The listing builds one solid part. Answer for the finished solid, in the listing's coordinates (mm). A direction names the side the tool comes from. Round coordinates to 2 decimals unless told otherwise and drop trailing zeros. Write each loop counter-clockwise with the first axis right and the second up, starting at its lowest first coordinate (ties: lowest second). Pieces come first, ordered by that corner, then holes. Notation, with made-up numbers: (-26.75, 82) - (17.25, 82) arc R19 ccw to (17.25, 99) - close; hole circle Ø9 at (-11.75, -31). An arc over 180 degrees is marked (long way). Return JSON: item names as keys, results as strings. Group by question number.
(1) Which of the six approach directions +Z, -Z, +X, -X, +Y, -Y give full straight-line access (tool end or side, diameter ignored) to faces 4 (the cylindrical face through (-17.281, 62.225, 6.084)), 5 (the flat face through (-20, -80, 7.9))?
(2) Section C-C, the plane x = -62 is taken. Write down the section's boundary in (y, z), then the cut area to 3 significant figures.
(3) Section B-B, the plane y = 30 is taken. Write down the section's boundary in (x, z), then the cut area to 3 significant figures.
(4) Section A-A, the plane z = 2.5 is taken. Give the number of separate pieces and of enclosed holes in the cut face, then the cut area to 3 significant figures.
(5) Each of these flat-tipped pins is pushed along its axis until it touches: pin 1 (1.5 mm diameter, centred on y = -48.5, z = 7.5, fed in from -X); pin 2 (5 mm diameter, centred on x = -19, z = 7, fed in from -Y); pin 3 (15 mm diameter, centred on x = -109.01, y = 9.57, fed in from +Z). Where does it stop, or does it pass through?
(6) Determine the mould class of faces 1 (the flat face through (-25, 8, 0)), 2 (the cylindrical face through (-22.908, 109.555, 5.916)), 3 (the cylindrical face through (51.5, 9.98, 9.04)) for opening direction Y: +Y half, -Y half, draft (parallel to the pull), parting line (faces both ways), or undercut.
(7) Find the intervals of material crossed by line 1 along X through (y, z) = (-79, 3.25); line 2 along X through (y, z) = (12, 3); line 3 along X through (y, z) = (-59, 6.5), in increasing order. Write a range as [from, to].
```python
from build123d import *

# Parameters (mm, degrees)
IZIM1_R                     = 4
Y_KSEKLIK_EKSTR_ZYON1_DEPTH = 12
IZIM2_R                     = 1.25
KES_EKSTR_ZYON1_DEPTH       = 50
KES_EKSTR_ZYON2_START       = -4.1
IZIM3_R                     = 10
IZIM3_R_2                   = 4
KES_EKSTR_ZYON2_DEPTH       = 4.1
KES_EKSTR_ZYON3_START       = -10
IZIM4_R                     = 1.35
IZIM4_R_2                   = 5.25
IZIM4_R_3                   = 4
KES_EKSTR_ZYON3_DEPTH       = 10
IZIM5_R                     = 9.5
KES_EKSTR_ZYON4_DEPTH       = 50
Y_KSEKLIK_EKSTR_ZYON2_START = -6
IZIM6_R                     = 9.5
IZIM6_R_2                   = 4.05
Y_KSEKLIK_EKSTR_ZYON2_DEPTH = 6
IZIM7_R                     = 2.6
KES_EKSTR_ZYON5_DEPTH       = 50


with BuildPart() as part:
    # Çizim1 → Yükseklik-Ekstrüzyon1 (new body)
    # profile 1 of 4: a face of its own
    with BuildSketch(Plane.XY):
        with BuildLine():
            Line((-24.007220217, 9.566787004), (-74.007220217, 59.566787004))
            ThreePointArc((-74.007220217, 59.566787004), (-124.007220217, 9.566787004), (-74.007220217, -40.433212996))
            Line((-74.007220217, -40.433212996), (-24.007220217, 9.566787004))
        make_face()
        with Locations((-109.007220217, 9.566787004)):
            Circle(IZIM1_R, mode=Mode.SUBTRACT)
    # profile 2 of 4: a face of its own
    with BuildSketch(Plane.XY):
        with BuildLine():
            ThreePointArc((25.992779783, 59.566787004), (-24.007220217, 109.566787004), (-74.007220217, 59.566787004))
            Line((-74.007220217, 59.566787004), (-24.007220217, 9.566787004))
            Line((-24.007220217, 9.566787004), (25.992779783, 59.566787004))
        make_face()
        with Locations((-24.007220217, 94.566787004)):
            Circle(IZIM1_R, mode=Mode.SUBTRACT)
    # profile 3 of 4: a face of its own
    with BuildSketch(Plane.XY):
        with BuildLine():
            Line((25.992779783, 59.566787004), (-24.007220217, 9.566787004))
            Line((-24.007220217, 9.566787004), (25.992779783, -40.433212996))
            ThreePointArc((25.992779783, -40.433212996), (75.992779783, 9.566787004), (25.992779783, 59.566787004))
        make_face()
        with Locations((60.992779783, 9.566787004)):
            Circle(IZIM1_R, mode=Mode.SUBTRACT)
    # profile 4 of 4: a face of its own
    with BuildSketch(Plane.XY):
        with BuildLine():
            Line((25.992779783, -40.433212996), (-24.007220217, 9.566787004))
            Line((-24.007220217, 9.566787004), (-74.007220217, -40.433212996))
            ThreePointArc((-74.007220217, -40.433212996), (-24.007220217, -90.433212996), (25.992779783, -40.433212996))
        make_face()
        with Locations((-24.007220217, -75.433212996)):
            Circle(IZIM1_R, mode=Mode.SUBTRACT)
    extrude(amount=Y_KSEKLIK_EKSTR_ZYON1_DEPTH)

    # Çizim2 → Kes-Ekstrüzyon1 (cut)
    with BuildSketch(Plane.XY.offset(12)):
        with Locations((-27.895001347, 40.325931985)):
            Circle(IZIM2_R)
        with Locations((-68.907194656, -0.686261324)):
            Circle(IZIM2_R)
        with Locations((-34.258962377, -35.334493602)):
            Circle(IZIM2_R)
        with Locations((6.753230931, 5.677699707)):
            Circle(IZIM2_R)
    extrude(amount=-KES_EKSTR_ZYON1_DEPTH, mode=Mode.SUBTRACT)

    # Çizim3 → Kes-Ekstrüzyon2 (cut)
    # profile 1 of 2: a face of its own
    with BuildSketch(Plane.XY.offset(12).offset(KES_EKSTR_ZYON2_START)):
        with Locations((-24.007220217, -75.433212996)):
            Circle(IZIM3_R)
        with Locations((-24.007220217, -75.433212996)):
            Circle(IZIM3_R_2, mode=Mode.SUBTRACT)
    # profile 2 of 2: a face of its own
    with BuildSketch(Plane.XY.offset(12).offset(KES_EKSTR_ZYON2_START)):
        with Locations((-24.007220217, 94.566787004)):
            Circle(IZIM3_R)
    extrude(amount=KES_EKSTR_ZYON2_DEPTH, mode=Mode.SUBTRACT)

    # Çizim4 → Kes-Ekstrüzyon3 (cut)
    # profile 1 of 11: a face of its own
    with BuildSketch(Plane.XY.offset(7.9).offset(KES_EKSTR_ZYON3_START)):
        with Locations((-26.880087777, -82.361173156)):
            Circle(IZIM4_R)
    # profile 2 of 11: a face of its own
    with BuildSketch(Plane.XY.offset(7.9).offset(KES_EKSTR_ZYON3_START)):
        with Locations((-17.079260057, -78.306080557)):
            Circle(IZIM4_R)
    # profile 3 of 11: a face of its own
    with BuildSketch(Plane.XY.offset(7.9).offset(KES_EKSTR_ZYON3_START)):
        with Locations((-30.935180377, -72.560345436)):
            Circle(IZIM4_R)
    # profile 4 of 11: a face of its own
    with BuildSketch(Plane.XY.offset(7.9).offset(KES_EKSTR_ZYON3_START)):
        with Locations((-21.134352656, -68.505252836)):
            Circle(IZIM4_R)
    # profile 5 of 11: a face of its own
    with BuildSketch(Plane.XY.offset(7.9).offset(KES_EKSTR_ZYON3_START)):
        with Locations((-24.007220217, -75.433212996)):
            Circle(IZIM4_R_2)
    # profile 6 of 11: a face of its own
    with BuildSketch(Plane.XY.offset(7.9).offset(KES_EKSTR_ZYON3_START)):
        with Locations((-21.134352656, 87.638826844)):
            Circle(IZIM4_R)
    # profile 7 of 11: a face of its own
    with BuildSketch(Plane.XY.offset(7.9).offset(KES_EKSTR_ZYON3_START)):
        with Locations((-30.935180377, 91.693919443)):
            Circle(IZIM4_R)
    # profile 8 of 11: a face of its own
    with BuildSketch(Plane.XY.offset(7.9).offset(KES_EKSTR_ZYON3_START)):
        with Locations((-24.007220217, 94.566787004)):
            Circle(IZIM4_R_2)
        with Locations((-24.007220217, 94.566787004)):
            Circle(IZIM4_R_3, mode=Mode.SUBTRACT)
    # profile 9 of 11: a face of its own
    with BuildSketch(Plane.XY.offset(7.9).offset(KES_EKSTR_ZYON3_START)):
        with Locations((-24.007220217, 94.566787004)):
            Circle(IZIM4_R_3)
    # profile 10 of 11: a face of its own
    with BuildSketch(Plane.XY.offset(7.9).offset(KES_EKSTR_ZYON3_START)):
        with Locations((-26.880087777, 101.494747164)):
            Circle(IZIM4_R)
    # profile 11 of 11: a face of its own
    with BuildSketch(Plane.XY.offset(7.9).offset(KES_EKSTR_ZYON3_START)):
        with Locations((-17.079260057, 97.439654564)):
            Circle(IZIM4_R)
    extrude(amount=KES_EKSTR_ZYON3_DEPTH, mode=Mode.SUBTRACT)

    # Çizim5 → Kes-Ekstrüzyon4 (cut)
    with BuildSketch(Plane.XY.offset(12)):
        with Locations((-109.007220217, 9.566787004)):
            Circle(IZIM5_R)
        with Locations((60.992779783, 9.566787004)):
            Circle(IZIM5_R)
    extrude(amount=-KES_EKSTR_ZYON4_DEPTH, mode=Mode.SUBTRACT)

    # Çizim6 → Yükseklik-Ekstrüzyon2 (add)
    # profile 1 of 2: a face of its own
    with BuildSketch(Plane(origin=(0, 0, 0), x_dir=(-1, 0, 0), z_dir=(0, 0, -1)).offset(Y_KSEKLIK_EKSTR_ZYON2_START)):
        with Locations(Location((109.007220217, 9.566787004, 0), (0, 0, 180))):
            Circle(IZIM6_R)
        with Locations((109.007220217, 9.566787004)):
            Circle(IZIM6_R_2, mode=Mode.SUBTRACT)
    # profile 2 of 2: a face of its own
    with BuildSketch(Plane(origin=(0, 0, 0), x_dir=(-1, 0, 0), z_dir=(0, 0, -1)).offset(Y_KSEKLIK_EKSTR_ZYON2_START)):
        with Locations(Location((-60.992779783, 9.566787004, 0), (0, 0, 180))):
            Circle(IZIM6_R)
        with Locations((-60.992779783, 9.566787004)):
            Circle(IZIM6_R_2, mode=Mode.SUBTRACT)
    extrude(amount=Y_KSEKLIK_EKSTR_ZYON2_DEPTH)

    # Çizim7 → Kes-Ekstrüzyon5 (cut)
    with BuildSketch(Plane.XY.offset(12)):
        with Locations((-16.717107836, 64.762736523)):
            Circle(IZIM7_R)
        with Locations((31.366153285, 16.679475402)):
            Circle(IZIM7_R)
        with Locations((-92.980015992, -11.500171633)):
            Circle(IZIM7_R)
        with Locations((-44.896754872, -59.583432754)):
            Circle(IZIM7_R)
    extrude(amount=-KES_EKSTR_ZYON5_DEPTH, mode=Mode.SUBTRACT)


solid = part.part
```
Working result:
{
 "1": {"face 4": "+Z, -Z", "face 5": "+Z"},
 "2": {"outline": "(-72.94, 0) - (92.07, 0) - (92.07, 12) - (-72.94, 12) - close", "area": "1,980 mm^2"},
 "3": {"outline": "(-119.64, 0) - (71.63, 0) - (71.63, 12) - (-119.64, 12) - close", "area": "2,300 mm^2"},
 "4": {"separate pieces": "1", "enclosed holes": "20", "area": "25,300 mm^2"},
 "5": {"pin 1": "stops at x = -73.47", "pin 2": "stops at y = -90.37", "pin 3": "stops at z = 6"},
 "6": {"face 1": "draft", "face 2": "+Y half", "face 3": "undercut"},
 "7": {"line 1": "x = [-55.83, -27.86], [-20.15, -18.24], [-15.92, 7.81]", "line 2": "x = [-123.95, -112.24], [-105.77, 57.76], [64.23, 75.93]", "line 3": "x = [-70.43, -47.43], [-42.36, 22.42]"}
}
